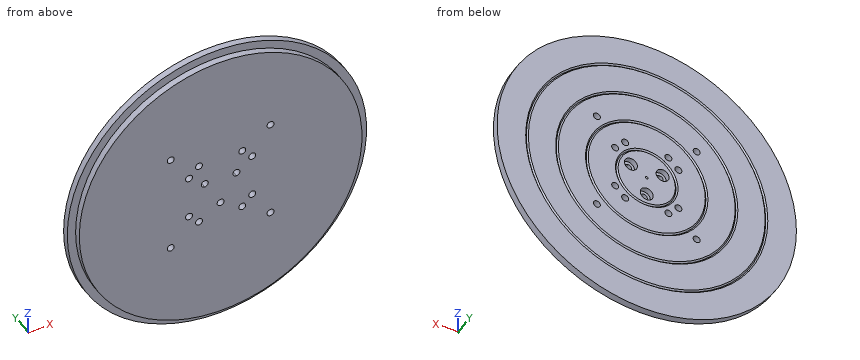
Autodesk Inventor part; units mm, degrees
ref_plane "YZ Plane" through (0, 0, 0) normal (1, 0, 0) x (0, 1, 0)
ref_plane "XZ Plane" through (0, 0, 0) normal (0, 1, 0) x (-1, 0, 0)
ref_plane "XY Plane" through (0, 0, 0) normal (0, 0, 1) x (1, 0, 0)
sketch "Sketch1" plane through (0, 0, 0) normal (0, 0, 1) x (1, 0, 0)
  line L0 (0, -1.6) -> (0, 9.6)
  line L1 (-108, 0) -> (18, 0)
  line L2 (0, 0) -> (-85, 0)
  line L3 (-85, 0) -> (-85, 4)
  line L4 (-85, 4) -> (-90, 4)
  line L5 (-90, 4) -> (-90, 8)
  line L6 (0, 7.2) -> (0, 0)
  line L7 (-0.8, 8) -> (0, 7.2)
  line L8 (-18.8, 8) -> (-18, 7.2)
  line L9 (-18, 7.2) -> (-17.2, 8)
  line L10 (-90, 8) -> (-18.8, 8) construction
  line L11 (-17.2, 8) -> (-0.8, 8)
  line L12 (-36.8, 8) -> (-36, 7.2)
  line L13 (-36, 7.2) -> (-35.2, 8)
  line L14 (-54.8, 8) -> (-54, 7.2)
  line L15 (-54, 7.2) -> (-53.2, 8)
  line L16 (-72.8, 8) -> (-72, 7.2)
  line L17 (-72, 7.2) -> (-71.2, 8)
  line L18 (-18.8, 8) -> (-35.2, 8)
  line L19 (-36.8, 8) -> (-53.2, 8)
  line L20 (-54.8, 8) -> (-71.2, 8)
  line L21 (-72.8, 8) -> (-90, 8)
  point P0 (-18, 8)
  point P1 (-36, 8)
  point P2 (-54, 8)
  point P3 (-72, 8)
  dimension "d2" = 5
  dimension "d3" = 4
  dimension "d4" = 90
  dimension "d7" = 18
  dimension "d11" = 18
  dimension "d17" = 8
  dimension "d18" = 135
  dimension "d19" = 0.8
revolve "Revolution1" add sketch "Sketch1" angle 360 about axis through (0, -10, 0) along (0, 1, 0)
sketch "Sketch2" plane through (0, 8, 0) normal (0, 1, 0) x (1, 0, 0)
  line L0 (-30, 30) -> (30, 30) construction
  line L1 (30, 30) -> (30, -30) construction
  line L2 (30, -30) -> (-30, -30) construction
  line L3 (-30, -30) -> (-30, 30) construction
  line L4 (-19, 13) -> (19, 13) construction
  line L5 (19, 13) -> (19, -13) construction
  line L6 (19, -13) -> (-19, -13) construction
  line L7 (-19, -13) -> (-19, 13) construction
  line L8 (-13, 19) -> (13, 19) construction
  line L9 (13, 19) -> (13, -19) construction
  line L10 (13, -19) -> (-13, -19) construction
  line L11 (-13, -19) -> (-13, 19) construction
  line L12 (0, 126) -> (0, -126)
  line L13 (-126, 0) -> (126, 0)
  circle A0 centre (0, 0) radius 11 construction
  point P0 (0, 11)
  point P1 (-9.5263, -5.5)
  point P2 (9.5263, -5.5)
  dimension "d21" = 60
  dimension "d22" = 26
  dimension "d23" = 38
  dimension "d25" = 22
  dimension "d26" = 120
  dimension "d27" = 120
hole "Hole1" at (0, 8, -11) at (-9.5263, 8, 5.5) at (9.5263, 8, 5.5) at (-30, 8, -30) at (-19, 8, -13) at (-13, 8, -19) at (13, 8, -19) at (19, 8, -13) at (30, 8, -30) at (30, 8, 30) at (-30, 8, 30) at (-13, 8, 19) at (13, 8, 19) at (19, 8, 13) at (-19, 8, 13) direction (0, -1, 0) diameter 4.2 end through all
hole "Hole2" at (0, 8, -11) direction (0, -1, 0) diameter 4.2 end through all counterbore diameter 7.8 counterbore depth 3.2
pattern_circular "Circular Pattern1" count 3 over 360 about axis through (0, -10, 0) along (0, 1, 0) of "Hole2"
properties part number "asztalv2"
Work out the finished part from the listing and answer in its coordinate system (mm). Coordinates: 2 decimals unless noted, no trailing zeros. Write each loop counter-clockwise with the first axis right and the second up, starting at its lowest first coordinate (ties: lowest second). Pieces come first, ordered by that corner, then holes. Notation, with made-up numbers: M 78.5,-4.75 L 133.5,-4.75 A14 ccw 133.5,3.25 Z; hole C 87.5,-6.5 d6. An arc over 180 degrees is marked long. Write item = value, one per line.
1. The part is cut by section A-A (z = 30). State how many separate pieces and enclosed holes the cut face has, then the cut area to 3 significant figures.
Solution:
separate_pieces = 3
enclosed_holes = 0
area = 1,240 mm2
2. The part is cut by section C-C (x = 76). Determine the outline of the cut face in (y, z).
Solution:
outline = M 0,-38.07 L 4,-38.07 L 4,-48.21 L 8,-48.21 L 8,48.21 L 4,48.21 L 4,38.07 L 0,38.07 Z
3. Flat-ended cylindrical pins translate along their axes: pin 1 (3 mm diameter, centred on y = 4.5, z = 59, fed in from +X); pin 2 (6 mm diameter, centred on x = 9.53, z = 5.5, fed in from -Y); pin 3 (2.5 mm diameter, centred on x = 7.5, z = 6, fed in from +Y); pin 4 (2.5 mm diameter, centred on x = 19, z = 13, fed in from +Y). Find the tip coordinate at first contact, or state that the pin passes through.
Solution:
pin_1 = 69.24
pin_2 = 0
pin_3 = 4.8
pin_4 = through
4. Straight lines are drawn through the part: line 1 (X direction, y = 4.5, z = 13); line 2 (Z direction, x = 0, y = 1.25); line 3 (X direction, y = 7.5, z = -55.5). For each, find the intervals that lie inside material, in ascending order. Write a range as from..to.
Solution:
line_1 = -89.06..-21.1, -16.9..16.9, 21.1..89.06
line_2 = -85..-13.1, -8.9..85
line_3 = -70.85..-46.34, -45.39..45.39, 46.34..70.85
